Check sheet for the modelled part. Datum: model origin and axes. Units: mm. A direction names the side the tool comes from. Round coordinates to 2 decimals unless told otherwise and drop trailing zeros. Order: outer loops, then holes, each group sorted by start corner. A loop starts at its lowest first (then second) coordinate and runs counter-clockwise, first axis right, second up. Notation, with made-up numbers: (37.25, -38) -> (60.25, -38) arc R26 ccw to (60.25, -14) -> close; hole circle Ø4 at (1.25, -32). An arc over 180 degrees is marked (long way). Answer in a Markdown table with one row per item. Add a question column.
1. Sectioned sample at D-D, the plane y = 9.25. Record the boundary of the cut face in (x, z), then the cut area to 3 significant figures.
2. Access from +Z, -Z, +X, -X, +Y, -Y to the whole of each face (thin tool, end or side, straight path). Record for faces 5 (the flat face through (-13, 6, 0)), 6 (the cylindrical face through (-14.443, 5.699, -4.715)), 7 (the cylindrical face through (8.715, 14.223, -4.699)), 8 (the cylindrical face through (18.727, 3.042, 0.358)).
3. Material ranges on L1, parallel to X at y = 3.05, z = 0; L2, parallel to X at y = 5.25, z = 1; L3, parallel to Y at x = 0, z = 2.5, recorded low to high. Write a range as from..to.
4. Sectioned sample at A-A, the plane x = -16. Record the boundary of the cut face in (y, z).
5. Draft check along Y on faces 1 (the cylindrical face through (1.846, 11.451, -0.056)), 2 (the conical face through (-1.73, 18.89, -0.04)), 3 (the flat face through (-2, 24, -1)), 4 (the cylindrical face through (20.715, 2.814, -4.699)). Enter one of: +Y half, -Y half, draft (parallel to the pull), parting line (faces both ways), or undercut.
6. Sectioned sample at B-B, the plane y = 21.75. Record the boundary of the cut face in (x, z), then the cut area to 3 significant figures.
7. Depth check by flat-ended pin: P1, Ø6, axis at y = 17, z = -3.5, coming from the -X side; P2, Ø0.6, axis at y = 4.5, z = 4.5, coming from the +X side; P3, Ø3, axis at x = 13, z = 3.5, coming from the +Y side. Enter the tip coordinate at first touch or a pass-through.
8. Sectioned sample at C-C, the plane x = -6.5. Record the boundary of the cut face in (y, z), then the cut area to 3 significant figures.
```python
from build123d import *

# Parameters (mm, degrees)
BOSS_EXTRUDE1_DEPTH      = 5
BOSS_EXTRUDE1_DEPTH_BACK = 5
CUT_EXTRUDE1_DEPTH       = 42
CUT_EXTRUDE1_DEPTH_BACK  = 42
SKETCH2_W                = 20
SKETCH2_H                = 16
CUT_EXTRUDE2_DEPTH       = 42
CUT_EXTRUDE2_DEPTH_BACK  = 42
SKETCH3_W                = 63
SKETCH3_H                = 20
BOSS_EXTRUDE2_DEPTH      = 24
CUT_EXTRUDE3_DEPTH       = 10
CUT_EXTRUDE3_DEPTH_BACK  = 10
CUT_EXTRUDE4_DEPTH       = 18
CUT_EXTRUDE4_DEPTH_BACK  = 18
SKETCH8_W                = 2.75
SKETCH8_H                = 6
SKETCH9_W                = 2.75
SKETCH9_H                = 6
SKETCH11_W               = 14
SKETCH11_H               = 8
CUT_EXTRUDE5_DEPTH       = 0.8


with BuildPart() as part:
    # Sketch1 → Boss-Extrude1 (new, two sides: drawn at the far end of the back side and taken through both)
    with BuildSketch(Plane.XY.offset(-BOSS_EXTRUDE1_DEPTH_BACK)):
        with BuildLine():
            Line((-21, 0), (21, 0))
            Line((21, 0), (21, 5))
            ThreePointArc((21, 5), (20.707106781, 5.707106781), (20, 6))
            Line((20, 6), (-20, 6))
            ThreePointArc((-20, 6), (-20.707106781, 5.707106781), (-21, 5))
            Line((-21, 5), (-21, 0))
        make_face()
    extrude(amount=BOSS_EXTRUDE1_DEPTH + BOSS_EXTRUDE1_DEPTH_BACK)

    # Sketch2 → Cut-Extrude1 (cut, two sides: drawn at the far end of the back side and taken through both)
    with BuildSketch(Plane(origin=(0, 0, 0), x_dir=(0, 0, -1), z_dir=(1, 0, 0)).offset(-CUT_EXTRUDE1_DEPTH_BACK)):
        with Locations((0, 3)):
            Rectangle(SKETCH2_W, SKETCH2_H)
        with BuildLine():
            Line((-5, 0), (5, 0))
            Line((5, 0), (5, 5))
            ThreePointArc((5, 5), (4.707106781, 5.707106781), (4, 6))
            Line((4, 6), (-4, 6))
            ThreePointArc((-4, 6), (-4.707106781, 5.707106781), (-5, 5))
            Line((-5, 5), (-5, 0))
        make_face(mode=Mode.SUBTRACT)
    extrude(amount=CUT_EXTRUDE1_DEPTH + CUT_EXTRUDE1_DEPTH_BACK, mode=Mode.SUBTRACT)

    # Sketch3 → Cut-Extrude2 (cut, two sides: drawn at the far end of the back side and taken through both)
    with BuildSketch(Plane(origin=(0, 0, 0), x_dir=(1, 0, 0), z_dir=(0, 1, 0)).offset(-CUT_EXTRUDE2_DEPTH_BACK)):
        Rectangle(SKETCH3_W, SKETCH3_H)
        with BuildLine():
            Line((-21, 4), (-21, -4))
            ThreePointArc((-21, -4), (-20.707106781, -4.707106781), (-20, -5))
            Line((-20, -5), (20, -5))
            ThreePointArc((20, -5), (20.707106781, -4.707106781), (21, -4))
            Line((21, -4), (21, 4))
            ThreePointArc((21, 4), (20.707106781, 4.707106781), (20, 5))
            Line((20, 5), (-20, 5))
            ThreePointArc((-20, 5), (-20.707106781, 4.707106781), (-21, 4))
        make_face(mode=Mode.SUBTRACT)
    extrude(amount=CUT_EXTRUDE2_DEPTH + CUT_EXTRUDE2_DEPTH_BACK, mode=Mode.SUBTRACT)

    # Sketch4 → Boss-Extrude2 (add)
    with BuildSketch(Plane(origin=(0, 0, 0), x_dir=(1, 0, 0), z_dir=(0, 1, 0))):
        with BuildLine():
            Line((-9, 4), (-9, -4))
            ThreePointArc((-9, -4), (-8.707106781, -4.707106781), (-8, -5))
            Line((-8, -5), (8, -5))
            ThreePointArc((8, -5), (8.707106781, -4.707106781), (9, -4))
            Line((9, -4), (9, 4))
            ThreePointArc((9, 4), (8.707106781, 4.707106781), (8, 5))
            Line((8, 5), (-8, 5))
            ThreePointArc((-8, 5), (-8.707106781, 4.707106781), (-9, 4))
        make_face()
    extrude(amount=BOSS_EXTRUDE2_DEPTH)

    # Sketch5 → Cut-Extrude3 (cut, two sides: drawn at the far end of the back side and taken through both)
    with BuildSketch(Plane.XY.offset(-CUT_EXTRUDE3_DEPTH_BACK)):
        with BuildLine():
            Line((-9, 48), (-9, 23))
            ThreePointArc((-9, 23), (-8.707106781, 23.707106781), (-8, 24))
            Line((-8, 24), (8, 24))
            ThreePointArc((8, 24), (8.707106781, 23.707106781), (9, 23))
            Line((9, 23), (9, 48))
            Line((9, 48), (-9, 48))
        make_face()
    extrude(amount=CUT_EXTRUDE3_DEPTH + CUT_EXTRUDE3_DEPTH_BACK, mode=Mode.SUBTRACT)

    # Sketch6 → Cut-Extrude4 (cut, two sides: drawn at the far end of the back side and taken through both)
    with BuildSketch(Plane(origin=(0, 0, 0), x_dir=(0, 0, -1), z_dir=(1, 0, 0)).offset(-CUT_EXTRUDE4_DEPTH_BACK)):
        with BuildLine():
            Line((-5, 48), (-5, 23))
            ThreePointArc((-5, 23), (-4.707106781, 23.707106781), (-4, 24))
            Line((-4, 24), (4, 24))
            ThreePointArc((4, 24), (4.707106781, 23.707106781), (5, 23))
            Line((5, 23), (5, 48))
            Line((5, 48), (-5, 48))
        make_face()
    extrude(amount=CUT_EXTRUDE4_DEPTH + CUT_EXTRUDE4_DEPTH_BACK, mode=Mode.SUBTRACT)

    # Sketch7 → Cut-Revolve1 (revolve, cut)
    with BuildSketch(Plane(origin=(0, 0, 0), x_dir=(0, 0, -1), z_dir=(1, 0, 0)), mode=Mode.PRIVATE) as cut_revolve1_sk:
        Polygon((-5, 15), (-5, 20), (-4, 19), (4, 19), (5, 20), (5, 15), align=None)
    revolve(cut_revolve1_sk.sketch.rotate(Axis((0, 15, -5), (0, 0, 1)), 270), axis=Axis((0, 15, -5), (0, 0, 1)), mode=Mode.SUBTRACT)

    # Sketch8 → Cut-Revolve2 (revolve, cut)
    with BuildSketch(Plane.XY, mode=Mode.PRIVATE) as cut_revolve2_sk:
        with Locations((-17.375, 3)):
            Rectangle(SKETCH8_W, SKETCH8_H)
    revolve(cut_revolve2_sk.sketch.rotate(Axis((-16, 6, 0), (0, -1, 0)), 90), axis=Axis((-16, 6, 0), (0, -1, 0)), mode=Mode.SUBTRACT)

    # Sketch9 → Cut-Revolve3 (revolve, cut)
    with BuildSketch(Plane.XY, mode=Mode.PRIVATE) as cut_revolve3_sk:
        with Locations((14.625, 3)):
            Rectangle(SKETCH9_W, SKETCH9_H)
    revolve(cut_revolve3_sk.sketch.rotate(Axis((16, 6, 0), (0, -1, 0)), 90), axis=Axis((16, 6, 0), (0, -1, 0)), mode=Mode.SUBTRACT)

    # Sketch10 → Cut-Revolve4 (revolve, cut)
    with BuildSketch(Plane.XY, mode=Mode.PRIVATE) as cut_revolve4_sk:
        Polygon((0, 24), (2, 24), (1.621, 23.621), (1.621, 19), (2, 18.621), (2, 15), (0, 15), align=None)
    revolve(cut_revolve4_sk.sketch.rotate(Axis((0, 15, 0), (0, 1, 0)), 270), axis=Axis((0, 15, 0), (0, 1, 0)), mode=Mode.SUBTRACT)

    # Sketch11 → Cut-Extrude5 (cut)
    with BuildSketch(Plane.XY.offset(5)):
        with Locations((0, 6)):
            Rectangle(SKETCH11_W, SKETCH11_H)
    extrude(amount=-CUT_EXTRUDE5_DEPTH, mode=Mode.SUBTRACT)


solid = part.part
```
Answer key:
| question | item | result |
|---|---|---|
| 1 | outline | (-9, -4) arc R1 ccw to (-8, -5) -> (8, -5) arc R1 ccw to (9, -4) -> (9, 4) arc R1 ccw to (8, 5) -> (7, 5) -> (7, 4.2) -> (-7, 4.2) -> (-7, 5) -> (-8, 5) arc R1 ccw to (-9, 4) -> close |
| 1 | area | 168 mm² |
| 2 | face 5 | +Z, -Z, -X, +Y |
| 2 | face 6 | -Z, -X, +Y |
| 2 | face 7 | -Z, +X, +Y |
| 2 | face 8 | +Y, -Y |
| 3 | L1 | x = -21..-18.75, -13.25..13.25, 18.75..21 |
| 3 | L2 | x = -20.97..-18.56, -13.44..13.44, 18.56..20.97 |
| 3 | L3 | y = 0..11, 19..24 |
| 4 | outline | (0, -5) -> (5, -5) arc R1 ccw to (6, -4) -> (6, -2.75) -> (0, -2.75) -> close; (0, 2.75) -> (6, 2.75) -> (6, 4) arc R1 ccw to (5, 5) -> (0, 5) -> close |
| 5 | face 1 | undercut |
| 5 | face 2 | undercut |
| 5 | face 3 | +Y half |
| 5 | face 4 | draft |
| 6 | outline | (-9, -4) arc R1 ccw to (-8, -5) -> (8, -5) arc R1 ccw to (9, -4) -> (9, 4) arc R1 ccw to (8, 5) -> (-8, 5) arc R1 ccw to (-9, 4) -> close; hole circle Ø3.24 at (0, 0) |
| 6 | area | 171 mm² |
| 7 | P1 | stops at x = -9 |
| 7 | P2 | stops at x = 20.98 |
| 7 | P3 | stops at y = 6 |
| 8 | outline | (0, -5) -> (23, -5) arc R1 ccw to (24, -4) -> (24, 4) arc R1 ccw to (23, 5) -> (10, 5) -> (10, 4.2) -> (2, 4.2) -> (2, 5) -> (0, 5) -> close |
| 8 | area | 233 mm² |
